from build123d import *

# Parameters (mm, degrees)
BOSS_EXTRUDE1_DEPTH             = 15
BOSS_EXTRUDE2_REACH             = 1239.023
BOSS_EXTRUDE2_DIRECTION_2_REACH = 1239.023
CUT_EXTRUDE2_DEPTH              = 1238.578280352
CUT_EXTRUDE2_DEPTH_BACK         = 1238.578280352
SKETCH5_W                       = 40
SKETCH5_H                       = 40
CUT_EXTRUDE3_DEPTH              = 1238.578280352
BOSS_EXTRUDE4_DEPTH             = 75
CUT_EXTRUDE4_DEPTH              = 1241.107934819
CUT_EXTRUDE4_DEPTH_BACK         = 1241.107934819
SKETCH8_W                       = 15
SKETCH8_H                       = 73.7
FILLET1_R                       = 5
CUT_EXTRUDE5_DEPTH              = 1241.107934819
CUT_EXTRUDE5_DEPTH_BACK         = 1241.107934819
SKETCH9_W                       = 1635
SKETCH9_H                       = 600
SKETCH10_W                      = 50
SKETCH10_H                      = 15
CUT_EXTRUDE6_DEPTH              = 126.494780768


with BuildPart() as part:
    # Sketch1 → Boss-Extrude1 (new body)
    with BuildSketch(Plane(origin=(0, 0, 0), x_dir=(1, 0, 0), z_dir=(0, 1, 0))):
        Polygon((-450, 300), (-400, 300), (-200, 250), (600, 40), (1200, 40), (1200, -40), (600, -40), (-200, -250), (-400, -300), (-450, -300), align=None)
    extrude(amount=BOSS_EXTRUDE1_DEPTH)

    # Boss-Extrude2: up to this face of the body (flat: up to its plane)
    boss_extrude2_end = Plane(part.part.faces().sort_by_distance((-425, 7.5, 300))[0])
    # Sketch2 → Boss-Extrude2 (add, up to the picked face)
    with BuildSketch(Plane.XY, mode=Mode.PRIVATE) as boss_extrude2_sk1:
        with BuildLine():
            Line((-425, 0), (-450, 0))
            Line((-450, 0), (-450, -40))
            Line((-450, -40), (-440, -40))
            Line((-440, -40), (-440, -15))
            ThreePointArc((-440, -15), (-435.606601718, -4.393398282), (-425, 0))
        make_face()
    boss_extrude2_tool1 = split(extrude(boss_extrude2_sk1.sketch, amount=BOSS_EXTRUDE2_REACH, mode=Mode.PRIVATE), bisect_by=boss_extrude2_end, keep=Keep.BOTH, mode=Mode.PRIVATE)
    # Sketch2 → Boss-Extrude2 (add, up to the picked face)
    with BuildSketch(Plane.XY, mode=Mode.PRIVATE) as boss_extrude2_sk2:
        with BuildLine():
            Line((-400, 0), (-425, 0))
            ThreePointArc((-425, 0), (-414.393398282, -4.393398282), (-410, -15))
            Line((-410, -15), (-410, -40))
            Line((-410, -40), (-400, -40))
            Line((-400, -40), (-400, 0))
        make_face()
    boss_extrude2_tool2 = split(extrude(boss_extrude2_sk2.sketch, amount=BOSS_EXTRUDE2_REACH, mode=Mode.PRIVATE), bisect_by=boss_extrude2_end, keep=Keep.BOTH, mode=Mode.PRIVATE)
    add(boss_extrude2_tool1.solids().sort_by(Axis((-444.100555, -18.206662, 0), (0, 0, 1)))[0])
    add(boss_extrude2_tool2.solids().sort_by(Axis((-405.899445, -18.206662, 0), (0, 0, 1)))[0])

    # Boss-Extrude2 direction 2: up to this face of the body (flat: up to its plane)
    boss_extrude2_direction_2_end = Plane(part.part.faces().sort_by_distance((-425, 7.5, -300))[0])
    # Sketch2 → Boss-Extrude2 direction 2 (add, up to the picked face)
    with BuildSketch(Plane.XY, mode=Mode.PRIVATE) as boss_extrude2_direction_2_sk1:
        with BuildLine():
            Line((-425, 0), (-450, 0))
            Line((-450, 0), (-450, -40))
            Line((-450, -40), (-440, -40))
            Line((-440, -40), (-440, -15))
            ThreePointArc((-440, -15), (-435.606601718, -4.393398282), (-425, 0))
        make_face()
    boss_extrude2_direction_2_tool1 = split(extrude(boss_extrude2_direction_2_sk1.sketch, amount=-BOSS_EXTRUDE2_DIRECTION_2_REACH, mode=Mode.PRIVATE), bisect_by=boss_extrude2_direction_2_end, keep=Keep.BOTH, mode=Mode.PRIVATE)
    # Sketch2 → Boss-Extrude2 direction 2 (add, up to the picked face)
    with BuildSketch(Plane.XY, mode=Mode.PRIVATE) as boss_extrude2_direction_2_sk2:
        with BuildLine():
            Line((-400, 0), (-425, 0))
            ThreePointArc((-425, 0), (-414.393398282, -4.393398282), (-410, -15))
            Line((-410, -15), (-410, -40))
            Line((-410, -40), (-400, -40))
            Line((-400, -40), (-400, 0))
        make_face()
    boss_extrude2_direction_2_tool2 = split(extrude(boss_extrude2_direction_2_sk2.sketch, amount=-BOSS_EXTRUDE2_DIRECTION_2_REACH, mode=Mode.PRIVATE), bisect_by=boss_extrude2_direction_2_end, keep=Keep.BOTH, mode=Mode.PRIVATE)
    add(boss_extrude2_direction_2_tool1.solids().sort_by(Axis((-444.100555, -18.206662, 0), (0, 0, -1)))[0])
    add(boss_extrude2_direction_2_tool2.solids().sort_by(Axis((-405.899445, -18.206662, 0), (0, 0, -1)))[0])

    # Sketch4 → Cut-Extrude2 (cut, two sides: drawn at the far end of the back side and taken through both)
    with BuildSketch(Plane(origin=(0, 0, 0), x_dir=(1, 0, 0), z_dir=(0, 1, 0)).offset(-CUT_EXTRUDE2_DEPTH_BACK)):
        Polygon((-450, 230), (-400, 230), (-150, 167.5), (-150, -167.5), (-400, -230), (-450, -230), align=None)
        Polygon((-100, 155), (-100, -155), (520, 0), align=None)
    extrude(amount=CUT_EXTRUDE2_DEPTH + CUT_EXTRUDE2_DEPTH_BACK, mode=Mode.SUBTRACT)

    # Sketch5 → Cut-Extrude3 (cut, through all)
    with BuildSketch(Plane(origin=(0, 0, 0), x_dir=(0, 0, -1), z_dir=(1, 0, 0))):
        with Locations((-265, -20)):
            Rectangle(SKETCH5_W, SKETCH5_H)
        with Locations((265, -20)):
            Rectangle(SKETCH5_W, SKETCH5_H)
    extrude(amount=-CUT_EXTRUDE3_DEPTH, mode=Mode.SUBTRACT)

    # Sketch7 → Boss-Extrude4 (add)
    with BuildSketch(Plane(origin=(1200, 0, 0), x_dir=(0, 0, -1), z_dir=(1, 0, 0))):
        with BuildLine():
            Line((-87.5, 50), (-40, 15))
            Line((-40, 15), (40, 15))
            Line((40, 15), (87.5, 50))
            Line((87.5, 50), (87.5, 88.7))
            Line((87.5, 88.7), (58.5, 88.7))
            Line((58.5, 88.7), (58.5, 63.2))
            Line((58.5, 63.2), (48.5, 63.2))
            Line((48.5, 63.2), (48.5, 88.7))
            Line((48.5, 88.7), (20, 88.7))
            Line((20, 88.7), (20, 50))
            ThreePointArc((20, 50), (0, 30), (-20, 50))
            Line((-20, 50), (-20, 88.7))
            Line((-20, 88.7), (-63, 88.7))
            Line((-63, 88.7), (-63, 63.2))
            Line((-63, 63.2), (-73, 63.2))
            Line((-73, 63.2), (-73, 88.7))
            Line((-73, 88.7), (-87.5, 88.7))
            Line((-87.5, 88.7), (-87.5, 50))
        make_face()
    extrude(amount=-BOSS_EXTRUDE4_DEPTH)

    # Sketch8 → Cut-Extrude4 (cut, two sides: drawn at the far end of the back side and taken through both)
    with BuildSketch(Plane.XY.offset(-CUT_EXTRUDE4_DEPTH_BACK)):
        with Locations((1147.5, 51.85)):
            Rectangle(SKETCH8_W, SKETCH8_H)
        with Locations((1177.5, 51.85)):
            Rectangle(SKETCH8_W, SKETCH8_H)
    extrude(amount=CUT_EXTRUDE4_DEPTH + CUT_EXTRUDE4_DEPTH_BACK, mode=Mode.SUBTRACT)

    # Fillet1
    fillet1_edges = [part.edges().sort_by_distance(p)[0] for p in [
        (1192.5, 50, 87.5),
        (1162.5, 50, 87.5),
        (1132.5, 50, 87.5),
        (1192.5, 50, -87.5),
        (1162.5, 50, -87.5),
        (1132.5, 50, -87.5),
        (1192.5, 88.7, -87.5),
        (1162.5, 88.7, -87.5),
        (1132.5, 88.7, -87.5),
        (1132.5, 88.7, -58.5),
        (1162.5, 88.7, -58.5),
        (1192.5, 88.7, -58.5),
        (1192.5, 88.7, -48.5),
        (1162.5, 88.7, -48.5),
        (1132.5, 88.7, -48.5),
        (1192.5, 88.7, -20),
        (1162.5, 88.7, -20),
        (1132.5, 88.7, -20),
        (1192.5, 88.7, 63),
        (1162.5, 88.7, 63),
        (1132.5, 88.7, 63),
        (1132.5, 88.7, 87.5),
        (1162.5, 88.7, 87.5),
        (1192.5, 88.7, 87.5),
        (1192.5, 88.7, 73),
        (1162.5, 88.7, 73),
        (1132.5, 88.7, 73),
        (1192.5, 88.7, 20),
        (1162.5, 88.7, 20),
        (1132.5, 88.7, 20),
        (600, 7.5, 40),
        (600, 7.5, -40),
        (520, 7.5, 0),
        (-440, -40, -292.5),
        (-440, -40, -237.5),
        (-400, -40, -292.5),
        (-400, -40, -237.5),
        (-450, -40, -237.5),
        (-410, -40, -237.5),
        (-450, -40, -292.5),
        (-410, -40, -292.5),
        (-150, 7.5, 167.5),
        (-100, 7.5, 155),
        (-150, 7.5, -167.5),
        (-100, 7.5, -155),
        (-450, -40, 237.5),
        (-410, -40, 237.5),
        (-440, -40, 237.5),
        (-400, -40, 237.5),
        (-450, -40, 292.5),
        (-440, -40, 292.5),
        (-400, -40, 292.5),
        (-410, -40, 292.5),
    ]]
    fillet(fillet1_edges, radius=FILLET1_R - 0.0001)  # a hair under: the kernel refuses the full size

    # Sketch9 → Cut-Extrude5 (cut, two sides: drawn at the far end of the back side and taken through both)
    with BuildSketch(Plane(origin=(0, 0, 0), x_dir=(1, 0, 0), z_dir=(0, 1, 0)).offset(-CUT_EXTRUDE5_DEPTH_BACK)):
        with Locations((367.5, 0)):
            Rectangle(SKETCH9_W, SKETCH9_H)
    extrude(amount=CUT_EXTRUDE5_DEPTH + CUT_EXTRUDE5_DEPTH_BACK, mode=Mode.SUBTRACT)

    # Sketch10 → Cut-Extrude6 (cut, through all)
    with BuildSketch(Plane(origin=(1200, 0, 0), x_dir=(0, 0, -1), z_dir=(1, 0, 0))):
        with Locations((0, 7.5)):
            Rectangle(SKETCH10_W, SKETCH10_H)
    extrude(amount=-CUT_EXTRUDE6_DEPTH, mode=Mode.SUBTRACT)


solid = part.part
Geometry check sheet. Reference: the model listing, model coordinates, mm. A direction names the side the tool comes from. Give positions to 0.01 mm unless a question says otherwise; leave off trailing zeros. Write each loop counter-clockwise with the first axis right and the second up, starting at its lowest first coordinate (ties: lowest second). Pieces come first, ordered by that corner, then holes. Notation, with made-up numbers: M -38,80 L 1,80 A14 cw 1,98 Z; hole C 21,36 d11. An arc over 180 degrees is marked long. Answer as CSV lines item,"result". Start each with the question number.
Q1. Go/stop test with flat-tipped pins: pin 1 (5 mm diameter, centred on x = 1194, y = 33, fed in from +Z); pin 2 (3 mm diameter, centred on x = 1190, z = 68.5, fed in from +Y); pin 3 (4.5 mm diameter, centred on x = 1193.5, y = 6.5, fed in from -Z). Record where each tip stops, or that it passes through.
Q2. Tool access check on faces 1 (the face through (1193, 73, -48.5)), 2 (the face through (1193, 88.7, 41)). Record the directions out of +Z, -Z, +X, -X, +Y, -Y that give a thin tool (end or side, any length) a straight path to the whole face; none if there is none.
Q3. Section check C-C, the plane z = 0. Record the cut outline in (x, y), then the cut area to 3 significant figures.
Q4. Section check B-B, the plane y = 44.5. Record the cut outline in (x, z), then the cut area to 3 significant figures.
Q5. Section check D-D, the plane y = 18.5. Record the cut outline in (x, z).
Q6. Release check for a two-part mould opening along Z. For faces 3 (the face through (1192.395, 50.242, -86.948)), 4 (the face through (1193, 74, -58.5)), 5 (the face through (1193, 0, -32)) record: pulls with the +Z half, pulls with the -Z half, needs draft (parallel to the pull), parting line crosses it, or undercut.
Q7. Material ranges on L1, parallel to Z at x = 1190.5, y = 68.5; L2, parallel to Z at x = 1198, y = 5.5; L3, parallel to Z at x = 1187, y = 57.5, recorded low to high.
Geometry says:
1,pin 1,"z = 67.82"
1,pin 2,"y = 63.2"
1,pin 3,"z = -40"
2,face 1,"+X, -X, +Y"
2,face 2,"+Z, -Z, +X, -X, +Y"
3,outline,"M 1185,15 L 1200,15 L 1200,30 L 1185,30 Z"
3,area,"225 mm^2"
4,outline,"M 1185,-80.04 L 1200,-80.04 L 1200,-19.23 L 1185,-19.23 Z; M 1185,19.23 L 1200,19.23 L 1200,80.04 L 1185,80.04 Z"
4,area,"1,820 mm^2"
5,outline,"M 1185,-44.75 L 1200,-44.75 L 1200,44.75 L 1185,44.75 Z"
6,face 3,"pulls with the -Z half"
6,face 4,"undercut"
6,face 5,"needs draft"
7,L1,"-87.5 to -58.5, -48.5 to -20, 20 to 63, 73 to 87.5"
7,L2,"-40 to -25, 25 to 40"
7,L3,"-87.5 to -20, 20 to 87.5"
